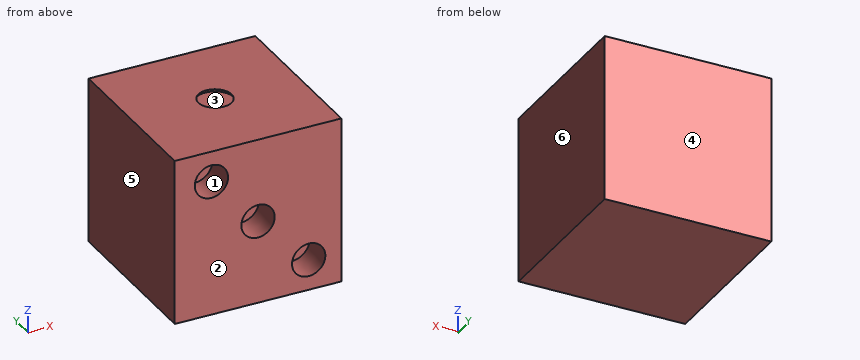
```python
from build123d import *

# Parameters (mm, degrees)
F0_W     = 25.4
F0_H     = 25.4
F1_DEPTH = 25.4
F2_R     = 2.54
F3_DEPTH = 0.508
F3_TAPER = -30
F4_R     = 2.54
F5_DEPTH = 5.08
F5_TAPER = -3


# Not quite as in the source:
# - the program builds the solid bodies; features that only make, move or delete a surface that nothing else refers to are left out


with BuildPart() as f1:
    # F0 (on Front) → F1 (new body)
    with BuildSketch(Plane.XZ):
        Rectangle(F0_W, F0_H)
    extrude(amount=F1_DEPTH)

    # F2 (on face) → F3 (cut)
    with BuildSketch(Plane.XY.offset(12.7)):
        with Locations((0, -12.7)):
            Circle(F2_R)
    extrude(amount=-F3_DEPTH, taper=F3_TAPER, mode=Mode.SUBTRACT)

    # F4 (on face) → F5 (cut)
    with BuildSketch(Plane.XZ.offset(25.4)):
        Circle(F4_R)
        with Locations((-7.1051362902, 8.0318916589)):
            Circle(F4_R)
        with Locations((7.7229747549, -8.0318916589)):
            Circle(F4_R)
    extrude(amount=-F5_DEPTH, taper=F5_TAPER, mode=Mode.SUBTRACT)


solid = f1.part
```
The listing builds one solid part. Answer for the finished solid, in the listing's coordinates (mm). Face numbers are marked on the shaded views. A direction names the side the tool comes from. Coordinates: 2 decimals unless noted, no trailing zeros. Loops run counter-clockwise (first coordinate to the right, second up) from the corner with the lowest first, then second, coordinate; pieces in that order, holes last. Notation, with made-up numbers: (48, -22.75) - (73, -22.75) arc R20 ccw to (73, -3.75) - close; hole circle Ø11 at (84.25, 27). An arc over 180 degrees is marked (long way). Write item = value, one per line.
1) Each of these flat-tipped pins is pushed along its axis until it touches: P1, Ø1.7, axis at x = 8.5, z = -7.5, coming from the -Y side; P2, Ø6, axis at x = -8, z = 7, coming from the -Y side; P3, Ø1.7, axis at x = 0.5, y = -12, coming from the +Z side. Where does it stop, or does it pass through?
Responses:
P1 = -20.32
P2 = -25.4
P3 = 12.19
2) Find the intervals of material crossed by line 1 along Y through (x, z) = (6.75, -8.25); line 2 along X through (y, z) = (-21, 9.75); line 3 along Z through (x, y) = (0.5, -22), in increasing order.
Responses:
line_1 = -20.32 to 0
line_2 = -12.7 to -9.28, -4.93 to 12.7
line_3 = -12.7 to -2.67, 2.67 to 12.7
3) Section A-A (x = 0) is taken. Determine the outline of the cut face in (y, z).
Responses:
outline = (-25.4, -12.7) - (0, -12.7) - (0, 12.7) - (-10.16, 12.7) - (-9.87, 12.19) - (-15.53, 12.19) - (-15.24, 12.7) - (-25.4, 12.7) - (-25.4, 2.54) - (-20.32, 2.81) - (-20.32, -2.81) - (-25.4, -2.54) - close
4) Section B-B (y = -20.75) is taken. Determine the outline of the cut face in (x, z), plus the area to 3 significant figures.
Responses:
outline = (-12.7, -12.7) - (12.7, -12.7) - (12.7, 12.7) - (-12.7, 12.7) - close; hole circle Ø5.57 at (-7.11, 8.03); hole circle Ø5.57 at (0, 0); hole circle Ø5.57 at (7.72, -8.03)
area = 572 mm^2
5) Determine the mould class of the marked faces 3, 4, 5 and 6 for opening direction X: pulls with the +X half, pulls with the -X half, needs draft (parallel to the pull), parting line crosses it, or undercut.
Responses:
face_3 = undercut
face_4 = needs draft
face_5 = pulls with the -X half
face_6 = pulls with the +X half
6) Which of the six approach directions +Z, -Z, +X, -X, +Y, -Y give full straight-line access (tool end or side, diameter ignored) to the marked faces 1 and 2?
Responses:
face_1 = none
face_2 = +Z, -Z, +X, -X, -Y
